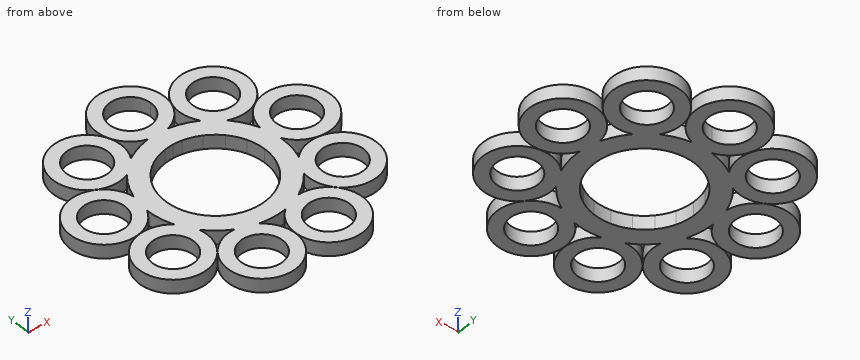
```python
from build123d import *

# Parameters (mm, degrees)
F0_R     = 4.6
F1_DEPTH = 3


with BuildPart() as f1:
    # F0 (on Top) → F1 (new body)
    with BuildSketch(Plane.XY):
        with BuildLine():
            ThreePointArc((8.426489, 7.070664), (7.070664, 8.426489), (5.5, 9.526279))
            ThreePointArc((5.5, 9.526279), (3.762222, 10.336619), (1.91013, 10.832885))
            ThreePointArc((1.91013, 10.832885), (0.958713, 10.958142), (0, 11))
            ThreePointArc((0, 11), (-0.958713, 10.958142), (-1.91013, 10.832885))
            ThreePointArc((-1.91013, 10.832885), (-3.762222, 10.336619), (-5.5, 9.526279))
            ThreePointArc((-5.5, 9.526279), (-7.070664, 8.426489), (-8.426489, 7.070664))
            ThreePointArc((-8.426489, 7.070664), (-9.526279, 5.5), (-10.336619, 3.762222))
            ThreePointArc((-10.336619, 3.762222), (-10.832885, 1.91013), (-11, 0))
            ThreePointArc((-11, 0), (-10.832885, -1.91013), (-10.336619, -3.762222))
            ThreePointArc((-10.336619, -3.762222), (-9.526279, -5.5), (-8.426489, -7.070664))
            ThreePointArc((-8.426489, -7.070664), (-7.070664, -8.426489), (-5.5, -9.526279))
            ThreePointArc((-5.5, -9.526279), (-3.762222, -10.336619), (-1.91013, -10.832885))
            ThreePointArc((-1.91013, -10.832885), (0, -11), (1.91013, -10.832885))
            ThreePointArc((1.91013, -10.832885), (3.762222, -10.336619), (5.5, -9.526279))
            ThreePointArc((5.5, -9.526279), (7.070664, -8.426489), (8.426489, -7.070664))
            ThreePointArc((8.426489, -7.070664), (9.526279, -5.5), (10.336619, -3.762222))
            ThreePointArc((10.336619, -3.762222), (10.832885, -1.91013), (11, 0))
            ThreePointArc((11, 0), (10.832885, 1.91013), (10.336619, 3.762222))
            ThreePointArc((10.336619, 3.762222), (9.526279, 5.5), (8.426489, 7.070664))
        make_face()
        with BuildLine():
            ThreePointArc((4.6, 22), (-3.252691, 25.252691), (0, 17.4))
            ThreePointArc((0, 17.4), (3.252691, 18.747309), (4.6, 22))
        make_face()
        with BuildLine():
            ThreePointArc((2.217213, 14.835227), (0, 29.5), (-2.217213, 14.835227))
            ThreePointArc((-2.217213, 14.835227), (-2.411174, 14.80494), (-2.604723, 14.772116))
            ThreePointArc((-2.604723, 14.772116), (-5.130302, 14.095389), (-7.5, 12.990381))
            ThreePointArc((-7.5, 12.990381), (-7.669365, 12.891115), (-7.837417, 12.78964))
            ThreePointArc((-7.837417, 12.78964), (-18.962234, 22.598311), (-11.234384, 9.939247))
            ThreePointArc((-11.234384, 9.939247), (-11.363498, 9.791369), (-11.490667, 9.641814))
            ThreePointArc((-11.490667, 9.641814), (-12.990381, 7.5), (-14.095389, 5.130302))
            ThreePointArc((-14.095389, 5.130302), (-14.161323, 4.945394), (-14.224832, 4.759638))
            ThreePointArc((-14.224832, 4.759638), (-29.051829, 5.122621), (-14.994862, 0.392582))
            ThreePointArc((-14.994862, 0.392582), (-14.998715, 0.196308), (-15, 0))
            ThreePointArc((-15, 0), (-14.772116, -2.604723), (-14.095389, -5.130302))
            ThreePointArc((-14.095389, -5.130302), (-14.027041, -5.314332), (-13.95629, -5.497451))
            ThreePointArc((-13.95629, -5.497451), (-25.547749, -14.75), (-11.739077, -9.337776))
            ThreePointArc((-11.739077, -9.337776), (-11.615867, -9.490608), (-11.490667, -9.641814))
            ThreePointArc((-11.490667, -9.641814), (-9.641814, -11.490667), (-7.5, -12.990381))
            ThreePointArc((-7.5, -12.990381), (-7.32935, -13.087422), (-7.157445, -13.182222))
            ThreePointArc((-7.157445, -13.182222), (-10.089594, -27.720932), (-2.990448, -14.698885))
            ThreePointArc((-2.990448, -14.698885), (-2.797825, -14.736763), (-2.604723, -14.772116))
            ThreePointArc((-2.604723, -14.772116), (0, -15), (2.604723, -14.772116))
            ThreePointArc((2.604723, -14.772116), (2.797825, -14.736763), (2.990448, -14.698885))
            ThreePointArc((2.990448, -14.698885), (10.089594, -27.720932), (7.157445, -13.182222))
            ThreePointArc((7.157445, -13.182222), (7.32935, -13.087422), (7.5, -12.990381))
            ThreePointArc((7.5, -12.990381), (9.641814, -11.490667), (11.490667, -9.641814))
            ThreePointArc((11.490667, -9.641814), (11.615867, -9.490608), (11.739077, -9.337776))
            ThreePointArc((11.739077, -9.337776), (25.547749, -14.75), (13.95629, -5.497451))
            ThreePointArc((13.95629, -5.497451), (14.027041, -5.314332), (14.095389, -5.130302))
            ThreePointArc((14.095389, -5.130302), (14.772116, -2.604723), (15, 0))
            ThreePointArc((15, 0), (14.998715, 0.196308), (14.994862, 0.392582))
            ThreePointArc((14.994862, 0.392582), (29.051829, 5.122621), (14.224832, 4.759638))
            ThreePointArc((14.224832, 4.759638), (14.161323, 4.945394), (14.095389, 5.130302))
            ThreePointArc((14.095389, 5.130302), (12.990381, 7.5), (11.490667, 9.641814))
            ThreePointArc((11.490667, 9.641814), (11.363498, 9.791369), (11.234384, 9.939247))
            ThreePointArc((11.234384, 9.939247), (18.962234, 22.598311), (7.837417, 12.78964))
            ThreePointArc((7.837417, 12.78964), (7.669365, 12.891115), (7.5, 12.990381))
            ThreePointArc((7.5, 12.990381), (5.130302, 14.095389), (2.604723, 14.772116))
            ThreePointArc((2.604723, 14.772116), (2.411174, 14.80494), (2.217213, 14.835227))
        make_face()
        with Locations((-7.524443, -20.673238)):
            Circle(F0_R, mode=Mode.SUBTRACT)
        with Locations((-19.052559, -11)):
            Circle(F0_R, mode=Mode.SUBTRACT)
        with Locations((7.524443, -20.673238)):
            Circle(F0_R, mode=Mode.SUBTRACT)
        with BuildLine():
            ThreePointArc((1.91013, 10.832885), (3.762222, 10.336619), (5.5, 9.526279))
            ThreePointArc((5.5, 9.526279), (7.070664, 8.426489), (8.426489, 7.070664))
            ThreePointArc((8.426489, 7.070664), (9.526279, 5.5), (10.336619, 3.762222))
            ThreePointArc((10.336619, 3.762222), (10.832885, 1.91013), (11, 0))
            ThreePointArc((11, 0), (10.832885, -1.91013), (10.336619, -3.762222))
            ThreePointArc((10.336619, -3.762222), (9.526279, -5.5), (8.426489, -7.070664))
            ThreePointArc((8.426489, -7.070664), (7.070664, -8.426489), (5.5, -9.526279))
            ThreePointArc((5.5, -9.526279), (3.762222, -10.336619), (1.91013, -10.832885))
            ThreePointArc((1.91013, -10.832885), (0, -11), (-1.91013, -10.832885))
            ThreePointArc((-1.91013, -10.832885), (-3.762222, -10.336619), (-5.5, -9.526279))
            ThreePointArc((-5.5, -9.526279), (-7.070664, -8.426489), (-8.426489, -7.070664))
            ThreePointArc((-8.426489, -7.070664), (-9.526279, -5.5), (-10.336619, -3.762222))
            ThreePointArc((-10.336619, -3.762222), (-10.832885, -1.91013), (-11, 0))
            ThreePointArc((-11, 0), (-10.832885, 1.91013), (-10.336619, 3.762222))
            ThreePointArc((-10.336619, 3.762222), (-9.526279, 5.5), (-8.426489, 7.070664))
            ThreePointArc((-8.426489, 7.070664), (-7.070664, 8.426489), (-5.5, 9.526279))
            ThreePointArc((-5.5, 9.526279), (-3.762222, 10.336619), (-1.91013, 10.832885))
            ThreePointArc((-1.91013, 10.832885), (-0.958713, 10.958142), (0, 11))
            ThreePointArc((0, 11), (0.958713, 10.958142), (1.91013, 10.832885))
        make_face(mode=Mode.SUBTRACT)
        with Locations((19.052559, -11)):
            Circle(F0_R, mode=Mode.SUBTRACT)
        with Locations((-21.665771, 3.82026)):
            Circle(F0_R, mode=Mode.SUBTRACT)
        with Locations((-14.141327, 16.852978)):
            Circle(F0_R, mode=Mode.SUBTRACT)
        with Locations((21.665771, 3.82026)):
            Circle(F0_R, mode=Mode.SUBTRACT)
        with BuildLine():
            ThreePointArc((4.6, 22), (3.252691, 18.747309), (0, 17.4))
            ThreePointArc((0, 17.4), (-3.252691, 25.252691), (4.6, 22))
        make_face(mode=Mode.SUBTRACT)
        with Locations((14.141327, 16.852978)):
            Circle(F0_R, mode=Mode.SUBTRACT)
    extrude(amount=F1_DEPTH)


solid = f1.part
```
Read the model definition and answer for the solid it produces. Units are mm, in the model's axes. Give positions to 0.01 mm unless a question says otherwise; leave off trailing zeros. Loops run counter-clockwise (first coordinate to the right, second up) from the corner with the lowest first, then second, coordinate; pieces in that order, holes last.
Item 1: The part is cut by section A-A (y = -24). Write down the section's boundary in (x, z), and give its area (3 significant figures).
Item 2: Each of these flat-tipped pins is pushed along its axis until it touches: pin 1 Ø5 at (x, y) = (-3.5, -16) entering from -Z; pin 2 Ø7.5 at (x, y) = (19.05, -11) entering from -Z. Where does it stop, or does it pass through?
Item 3: Find the intervals of material crossed by line 1 along X through (y, z) = (1.5, 0.95); line 2 along X through (y, z) = (4, 2); line 3 along X through (y, z) = (7, 2.6), in increasing order.
Item 4: The part is cut by section D-D (z = 0.55). Give the number of separate pieces and of enclosed holes in the cut face, and give its area (3 significant figures).
Item 5: The part is cut by section C-C (x = 20). Write down the section's boundary in (y, z), and give its area (3 significant figures).
Item 6: The part is cut by section B-B (x = -13). Write down the section's boundary in (y, z), and give its area (3 significant figures).
Taken from the geometry:
1. outline: (-14.25, 0) - (-10.7, 0) - (-10.7, 3) - (-14.25, 3) - close; (-4.35, 0) - (-0.8, 0) - (-0.8, 3) - (-4.35, 3) - close; (0.8, 0) - (4.35, 0) - (4.35, 3) - (0.8, 3) - close; (10.7, 0) - (14.25, 0) - (14.25, 3) - (10.7, 3) - close
1. area: 42.5 mm2
2. pin 1: stops at z = 0
2. pin 2: passes through
3. line 1: x = -28.8 to -25.64, -17.69 to -10.9, 10.9 to 17.69, 25.64 to 28.8
3. line 2: x = -29.16 to -26.26, -17.07 to -10.25, 10.25 to 17.07, 26.26 to 29.16
3. line 3: x = -28.46 to -24.99, -18.34 to -14.87, -13.27 to -8.49, 8.49 to 13.27, 14.87 to 18.34, 24.99 to 28.46
4. separate pieces: 1
4. enclosed holes: 10
4. area: 1,310 mm2
5. outline: (-18.44, 0) - (-15.5, 0) - (-15.5, 3) - (-18.44, 3) - close; (-6.5, 0) - (-3.56, 0) - (-3.56, 3) - (-6.5, 3) - close; (-3.49, 0) - (-0.47, 0) - (-0.47, 3) - (-3.49, 3) - close; (8.11, 0) - (11.13, 0) - (11.13, 3) - (8.11, 3) - close; (12.17, 0) - (21.54, 0) - (21.54, 3) - (12.17, 3) - close
5. area: 63.9 mm2
6. outline: (-25.8, 0) - (-15.55, 0) - (-15.55, 3) - (-25.8, 3) - close; (-15.43, 0) - (7.48, 0) - (7.48, 3) - (-15.43, 3) - close; (9.44, 0) - (12.4, 0) - (12.4, 3) - (9.44, 3) - close; (21.31, 0) - (24.27, 0) - (24.27, 3) - (21.31, 3) - close
6. area: 117 mm2
